from build123d import *

# Parameters (mm, degrees)
SKETCH1_W           = 177.8
SKETCH1_H           = 76.2
SKETCH1_R           = 2.5527
SKETCH1_R_2         = 4.1275
SKETCH1_R_3         = 19.177
BOSS_EXTRUDE1_DEPTH = 3.175
SKETCH2_W           = 3.175
SKETCH2_H           = 76.2
BOSS_EXTRUDE2_DEPTH = 19.05
SKETCH3_R           = 2.54
CUT_EXTRUDE1_DEPTH  = 197.11331534


with BuildPart() as part:
    # Sketch1 → Boss-Extrude1 (new body)
    with BuildSketch(Plane.XY):
        with Locations((51.430541204, 41.609734844)):
            Rectangle(SKETCH1_W, SKETCH1_H)
        with Locations((89.530541204, 9.859734844)):
            Circle(SKETCH1_R, mode=Mode.SUBTRACT)
        with Locations((89.530541204, 73.359734844)):
            Circle(SKETCH1_R, mode=Mode.SUBTRACT)
        with Locations((-12.069458796, 73.359734844)):
            Circle(SKETCH1_R, mode=Mode.SUBTRACT)
        with Locations((-12.069458796, 64.427395008)):
            Circle(SKETCH1_R, mode=Mode.SUBTRACT)
        with Locations((38.730541204, 73.359734844)):
            Circle(SKETCH1_R, mode=Mode.SUBTRACT)
        with Locations((35.301541204, 64.427395008)):
            Circle(SKETCH1_R, mode=Mode.SUBTRACT)
        with Locations((9.774192889, 51.727395008)):
            Circle(SKETCH1_R, mode=Mode.SUBTRACT)
        with Locations((19.299192889, 42.202395008)):
            Circle(SKETCH1_R, mode=Mode.SUBTRACT)
        with Locations((-12.069458796, 20.433674276)):
            Circle(SKETCH1_R, mode=Mode.SUBTRACT)
        with Locations((35.301541204, 20.433674276)):
            Circle(SKETCH1_R, mode=Mode.SUBTRACT)
        with Locations((38.730541204, 9.859734844)):
            Circle(SKETCH1_R, mode=Mode.SUBTRACT)
        with Locations((55.695028962, 24.33315969)):
            Circle(SKETCH1_R, mode=Mode.SUBTRACT)
        with Locations((55.695028962, 60.254184174)):
            Circle(SKETCH1_R_2, mode=Mode.SUBTRACT)
        with Locations((91.616053446, 60.254184174)):
            Circle(SKETCH1_R, mode=Mode.SUBTRACT)
        with Locations((91.616053446, 24.33315969)):
            Circle(SKETCH1_R_2, mode=Mode.SUBTRACT)
        with Locations((73.655541204, 42.202395008)):
            Circle(SKETCH1_R_3, mode=Mode.SUBTRACT)
        with Locations((-12.069458796, 9.859734844)):
            Circle(SKETCH1_R, mode=Mode.SUBTRACT)
        with Locations((121.280541204, 42.202395008)):
            Circle(SKETCH1_R, mode=Mode.SUBTRACT)
    extrude(amount=BOSS_EXTRUDE1_DEPTH)

    # Sketch2 → Boss-Extrude2 (add)
    with BuildSketch(Plane.XY.offset(3.175)):
        with Locations((-35.881958796, 41.609734844)):
            Rectangle(SKETCH2_W, SKETCH2_H)
        with Locations((138.743041204, 41.609734844)):
            Rectangle(SKETCH2_W, SKETCH2_H)
    extrude(amount=BOSS_EXTRUDE2_DEPTH)

    # Sketch3 → Cut-Extrude1 (cut, through all)
    with BuildSketch(Plane(origin=(140.330541204, 0, 0), x_dir=(0, 0, -1), z_dir=(1, 0, 0))):
        with Locations((-12.7, 35.259734844)):
            Circle(SKETCH3_R)
        with Locations((-12.7, 22.559734844)):
            Circle(SKETCH3_R)
        with Locations((-12.7, 9.859734844)):
            Circle(SKETCH3_R)
    extrude(amount=-CUT_EXTRUDE1_DEPTH, mode=Mode.SUBTRACT)


solid = part.part
Read the model definition and answer for the solid it produces. Units are mm, in the model's axes. A direction names the side the tool comes from. Round coordinates to 2 decimals unless told otherwise and drop trailing zeros. Write each loop counter-clockwise with the first axis right and the second up, starting at its lowest first coordinate (ties: lowest second). Pieces come first, ordered by that corner, then holes.
1. The part is cut by section C-C, the plane x = 98.5. Determine the outline of the cut face in (y, z) (3 decimals), then the cut area to 3 significant figures.
2. The part is cut by section A-A, the plane z = 12.7. State how many separate pieces and enclosed holes the cut face has, then the cut area to 3 significant figures.
3. Straight lines are drawn through the part: L1, parallel to X at y = 67, z = 17; L2, parallel to Z at x = 37.5, y = 15 (3 decimals); L3, parallel to Y at x = 86.5, z = 1.5. For each, find the intervals that lie inside material, in ascending order.
4. Determine the mould class of faces 1 (the face through (-37.469, 41, 11)), 2 (the face through (-35.86, 8.314, 14.716)), 3 (the face through (18.967, 44.733, 1.565)) for opening direction X: pulls with the +X half, pulls with the -X half, needs draft (parallel to the pull), parting line crosses it, or undercut.
5. Which of the six approach directions +Z, -Z, +X, -X, +Y, -Y give full straight-line access (tool end or side, diameter ignored) to faces 4 (the face through (34.97, 66.96, 1.57)), 5 (the face through (50, 42, 3.175))?
6. The part is cut by section B-B, the plane z = 5. Determine the outline of the cut face in (x, y), then the cut area to 3 significant figures.
7. Given pin 1 Ø4.5 at (x, y) = (-12.07, 73.36) entering from +Z; pin 2 Ø6.5 at (x, y) = (-12.07, 64.43) entering from +Z (3 decimals), each flat-ended and moving along its own axis, determine where each tip first touches the part or whether it passes through.
Values:
1. outline: (3.51, 0) - (79.71, 0) - (79.71, 3.175) - (3.51, 3.175) - close
1. area: 242 mm2
2. separate pieces: 8
2. enclosed holes: 0
2. area: 387 mm2
3. L1: x = -37.47 to -34.29, 137.16 to 140.33
3. L2: z = 0 to 3.175
3. L3: y = 3.51 to 27.96, 56.44 to 79.71
4. face 1: pulls with the -X half
4. face 2: needs draft
4. face 3: undercut
5. face 4: +Z, -Z
5. face 5: +Z, +Y, -Y
6. outline: (-37.47, 3.51) - (-34.29, 3.51) - (-34.29, 79.71) - (-37.47, 79.71) - close; (137.16, 3.51) - (140.33, 3.51) - (140.33, 79.71) - (137.16, 79.71) - close
6. area: 484 mm2
7. pin 1: passes through
7. pin 2: stops at z = 3.175
